Verification items for the finished model (mm, model axes). Round coordinates to 2 decimals unless told otherwise and drop trailing zeros. Order: outer loops, then holes, each group sorted by start corner. A loop starts at its lowest first (then second) coordinate and runs counter-clockwise, first axis right, second up. Notation, with made-up numbers: (4, -8.75) -> (38, -8.75) arc R10 ccw to (38, 4.25) -> close; hole circle Ø9 at (3.5, 64). An arc over 180 degrees is marked (long way). Return JSON: item names as keys, results as strings. Group by question number.
1) Depth check by flat-ended pin: pin 1 (7 mm diameter, centred on y = 5, z = -143.5, fed in from -X); pin 2 (1.9 mm diameter, centred on y = 6, z = -7, fed in from -X); pin 3 (5 mm diameter, centred on x = 124.26, y = 9.325, fed in from +Z); pin 4 (6.5 mm diameter, centred on x = 68, y = 7, fed in from -Z). Enter the tip coordinate at first touch or a pass-through.
2) Section check C-C on z = -45. Enter the section's corners in (x, y) (3 decimals).
3) Section check D-D on x = 95. Enter the section's corners in (y, z) (3 decimals), plus the area to 3 significant figures.
4) Section check A-A on x = 124.26. Enter the section's corners in (y, z) (3 decimals), plus the area to 3 significant figures.
5) Scan lines: L1, parallel to Y at x = 124, z = -144; L2, parallel to Y at x = 7, z = -43 (3 decimals); L3, parallel to Z at x = 127, y = 5.5. Record each from-to range of solid material in increasing order.
6) Section check B-B on x = 29. Enter the section's corners in (y, z) (3 decimals).
```python
from build123d import *

# Parameters (mm, degrees)
SKETCH1_W           = 139.5
SKETCH1_H           = 152.4
BOSS_EXTRUDE1_DEPTH = 6.35
SKETCH2_W           = 139.5
SKETCH2_H           = 152.4
CUT_EXTRUDE1_DEPTH  = 3.375
SKETCH3_R           = 3.175
BOSS_EXTRUDE2_DEPTH = 12.7
SKETCH4_R           = 3.175000001
SKETCH4_R_2         = 3.175
BOSS_EXTRUDE3_DEPTH = 12.7
SKETCH5_R           = 7.62
CUT_EXTRUDE2_DEPTH  = 16.675000317


with BuildPart() as part:
    # Sketch1 → Boss-Extrude1 (new body)
    with BuildSketch(Plane(origin=(0, 0, 0), x_dir=(1, 0, 0), z_dir=(0, 1, 0))):
        with Locations((69.75, 76.2)):
            Rectangle(SKETCH1_W, SKETCH1_H)
    extrude(amount=BOSS_EXTRUDE1_DEPTH)

    # Sketch2 → Cut-Extrude1 (cut)
    with BuildSketch(Plane(origin=(0, 6.35, 0), x_dir=(1, 0, 0), z_dir=(0, 1, 0))):
        with Locations((69.75, 76.2)):
            Rectangle(SKETCH2_W, SKETCH2_H)
    extrude(amount=-CUT_EXTRUDE1_DEPTH, mode=Mode.SUBTRACT)

    # Sketch3 → Boss-Extrude2 (add)
    with BuildSketch(Plane.XY):
        with BuildLine():
            Line((63.4, 9.325), (63.4, 2.975))
            Line((63.4, 2.975), (76.1, 2.975))
            Line((76.1, 2.975), (76.1, 9.325000633))
            ThreePointArc((76.1, 9.325000633), (69.749999683, 15.675000317), (63.4, 9.325))
        make_face()
        with Locations((69.75, 9.325000317)):
            Circle(SKETCH3_R, mode=Mode.SUBTRACT)
    extrude(amount=-BOSS_EXTRUDE2_DEPTH)

    # Sketch4 → Boss-Extrude3 (add)
    with BuildSketch(Plane(origin=(0, 0, -152.4), x_dir=(-1, 0, 0), z_dir=(0, 0, -1))):
        with BuildLine():
            Line((-130.61, 9.325), (-130.61, 2.975))
            Line((-130.61, 2.975), (-117.91, 2.975))
            Line((-117.91, 2.975), (-117.91, 9.325))
            ThreePointArc((-117.91, 9.325), (-124.26, 15.675), (-130.61, 9.325))
        make_face()
        with Locations((-124.26, 9.325)):
            Circle(SKETCH4_R, mode=Mode.SUBTRACT)
        with BuildLine():
            Line((-21.59, 9.325), (-21.59, 2.975))
            Line((-21.59, 2.975), (-8.89, 2.975))
            Line((-8.89, 2.975), (-8.89, 9.325))
            ThreePointArc((-8.89, 9.325), (-15.24, 15.675), (-21.59, 9.325))
        make_face()
        with Locations((-15.24, 9.325)):
            Circle(SKETCH4_R_2, mode=Mode.SUBTRACT)
    extrude(amount=-BOSS_EXTRUDE3_DEPTH)

    # Sketch5 → Cut-Extrude2 (cut, through all)
    with BuildSketch(Plane.XZ):
        with Locations((33.274, -136.991598)):
            Circle(SKETCH5_R)
    extrude(amount=-CUT_EXTRUDE2_DEPTH, mode=Mode.SUBTRACT)


solid = part.part
```
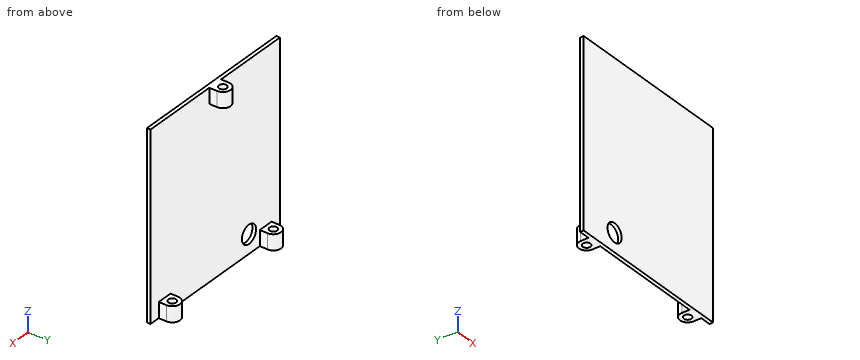
Check result:
{
 "1": {"pin 1": "x = 0", "pin 2": "x = 63.4", "pin 3": "through", "pin 4": "z = -12.7"},
 "2": {"outline": "(0, 0) -> (139.5, 0) -> (139.5, 2.975) -> (0, 2.975) -> close"},
 "3": {"outline": "(0, -152.4) -> (2.975, -152.4) -> (2.975, 0) -> (0, 0) -> close", "area": "453 mm^2"},
 "4": {"outline": "(0, -152.4) -> (6.15, -152.4) -> (6.15, -139.7) -> (2.975, -139.7) -> (2.975, 0) -> (0, 0) -> close; (12.5, -152.4) -> (15.675, -152.4) -> (15.675, -139.7) -> (12.5, -139.7) -> close", "area": "534 mm^2"},
 "5": {"L1": "0 to 6.16, 12.49 to 15.67", "L2": "0 to 2.975", "L3": "-152.4 to -139.7"},
 "6": {"outline": "(0, -152.4) -> (2.975, -152.4) -> (2.975, -143.3) -> (0, -143.3) -> close; (0, -130.683) -> (2.975, -130.683) -> (2.975, 0) -> (0, 0) -> close"}
}
